Design review of the part built by this model. Coordinates are the model's own, in mm. Round coordinates to 2 decimals unless told otherwise and drop trailing zeros. Loops run counter-clockwise (first coordinate to the right, second up) from the corner with the lowest first, then second, coordinate; pieces in that order, holes last. Notation, with made-up numbers: (-38, -10) - (-10, -10) arc R19 cw to (-10, 0) - close; hole circle Ø5 at (-3.75, 24). An arc over 180 degrees is marked (long way). Answer as CSV lines item,"result". Start each with the question number.
(1) For P1, Ø4, axis at x = -32.34, y = 13.39, coming from the -Z side, flat-tipped, find the tip position at first contact; note if it passes through.
(2) Consider section C-C (x = -10.5). Give the boundary of the cut face in (y, z).
(3) Consider section D-D (z = 13.1). Count the separate pieces of the cut face and the enclosed holes in it, and give its area (3 significant figures).
(4) Wall thickness on L1, parallel to Y at x = -0.5, z = 12.3; L2, parallel to X at y = -2, z = 12.2; L3, parallel to Y at x = -6.5, z = 12.65: over which ranges is each line inside the solid? List them lowest first.
(5) Consider section A-A (x = 0). Give the boundary of the cut face in (y, z), and give its area (3 significant figures).
from build123d import *

# Parameters (mm, degrees)
SKETCH_1_R          = 40
EXTRUDE_1_DEPTH     = 12
SKETCH_8_R          = 45
EXTRUDE_3_DEPTH     = 2
SKETCH_2_R          = 7.5
CUT_EXTRUDE_1_DEPTH = 66.161338231
HOLE_WIZARD_M31_D   = 3.4
HOLE_WIZARD_M32_D   = 3.4
SKETCH_10_R         = 7.5
CUT_EXTRUDE_2_DEPTH = 66.161338231
HOLE_WIZARD_M33_D   = 3.4
SKETCH_17_R         = 17
CUT_EXTRUDE_3_DEPTH = 1.5
SKETCH_18_R         = 44.163841719
CUT_EXTRUDE_4_DEPTH = 12
SKETCH_19_R         = 17.5
CUT_EXTRUDE_5_DEPTH = 64.671029519


with BuildPart() as part:
    # Эскиз1 → Бобышка-Вытянуть1 (new body)
    with BuildSketch(Plane.XY):
        Circle(SKETCH_1_R)
    extrude(amount=EXTRUDE_1_DEPTH)

    # Эскиз8 → Бобышка-Вытянуть3 (add)
    with BuildSketch(Plane.XY.offset(12)):
        Circle(SKETCH_8_R)
    extrude(amount=EXTRUDE_3_DEPTH)

    # Эскиз2 → Вырез-Вытянуть1 (cut, through all)
    with BuildSketch(Plane(origin=(0, 0, 14), x_dir=(-1, 0, 0), z_dir=(0, 0, -1))):
        Circle(SKETCH_2_R)
    extrude(amount=CUT_EXTRUDE_1_DEPTH, mode=Mode.SUBTRACT)

    # Отверстие с зазором M31 (through all)
    with Locations(Plane(origin=(-6.663493146, -3.889871465, 14), x_dir=(-1, 0, 0), z_dir=(0, 0, 1))):
        with Locations((20.599623529, -37.010635762)):
            Hole(HOLE_WIZARD_M31_D / 2)

    # Отверстие с зазором M32 (through all)
    with Locations(Plane.XY.offset(14)):
        with Locations((0, 12.5), (-12.5, 0), (0, -12.5), (12.5, 0)):
            Hole(HOLE_WIZARD_M32_D / 2)

    # Эскиз10 → Вырез-Вытянуть2 (cut, through all)
    with BuildSketch(Plane(origin=(0, 0, 0), x_dir=(-1, 0, 0), z_dir=(0, 0, -1))):
        with Locations((0, 27.5)):
            Circle(SKETCH_10_R)
        with Locations((19.445436483, 19.445436483)):
            Circle(SKETCH_10_R)
        with Locations((27.5, 0)):
            Circle(SKETCH_10_R)
        with Locations((19.445436483, -19.445436483)):
            Circle(SKETCH_10_R)
        with Locations((0, -27.5)):
            Circle(SKETCH_10_R)
        with Locations((-19.445436483, -19.445436483)):
            Circle(SKETCH_10_R)
        with Locations((-27.5, 0)):
            Circle(SKETCH_10_R)
        with Locations((-19.445436483, 19.445436483)):
            Circle(SKETCH_10_R)
    extrude(amount=-CUT_EXTRUDE_2_DEPTH, mode=Mode.SUBTRACT)

    # Отверстие с зазором M33 (through all)
    with Locations(Plane(origin=(0, 0, 0), x_dir=(-1, 0, 0), z_dir=(0, 0, -1))):
        with Locations((-13.393920133, 32.335783638), (13.393920133, -32.335783638), (32.335783638, 13.393920133), (-32.335783638, -13.393920133)):
            Hole(HOLE_WIZARD_M33_D / 2)

    # Эскиз17 → Вырез-Вытянуть3 (cut)
    with BuildSketch(Plane(origin=(0, 0, 0), x_dir=(-1, 0, 0), z_dir=(0, 0, -1))):
        Circle(SKETCH_17_R)
    extrude(amount=-CUT_EXTRUDE_3_DEPTH, mode=Mode.SUBTRACT)

    # Эскиз18 → Вырез-Вытянуть4 (cut)
    with BuildSketch(Plane(origin=(0, 0, 0), x_dir=(-1, 0, 0), z_dir=(0, 0, -1))):
        Circle(SKETCH_18_R)
    extrude(amount=-CUT_EXTRUDE_4_DEPTH, mode=Mode.SUBTRACT)

    # Эскиз19 → Вырез-Вытянуть5 (cut, through all)
    with BuildSketch(Plane(origin=(0, 0, 12), x_dir=(-1, 0, 0), z_dir=(0, 0, -1))):
        Circle(SKETCH_19_R)
    extrude(amount=-CUT_EXTRUDE_5_DEPTH, mode=Mode.SUBTRACT)


solid = part.part
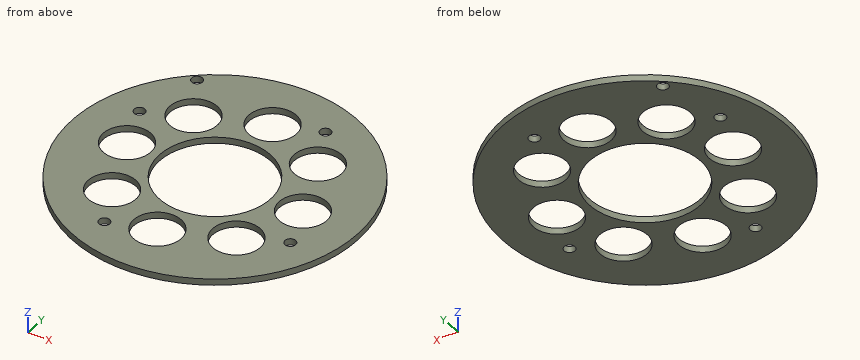
Determined:
1,P1,"stops at z = 12"
2,outline,"(-43.76, 12) - (-14, 12) - (-14, 14) - (-43.76, 14) - close; (14, 12) - (43.76, 12) - (43.76, 14) - (14, 14) - close"
3,separate pieces,"1"
3,enclosed holes,"14"
3,area,"3,940 mm^2"
4,L1,"y = -45 to -34.98, -20.02 to -17.49, 17.49 to 20.02, 34.98 to 45"
4,L2,"x = -44.96 to -34.73, -20.27 to -17.39, 17.39 to 20.27, 34.73 to 44.96"
4,L3,"y = -44.53 to -31.24, -23.76 to -16.25, 16.25 to 23.76, 31.24 to 44.53"
5,outline,"(-45, 12) - (-35, 12) - (-35, 14) - (-45, 14) - close; (-20, 12) - (-17.5, 12) - (-17.5, 14) - (-20, 14) - close; (17.5, 12) - (20, 12) - (20, 14) - (17.5, 14) - close; (35, 12) - (45, 12) - (45, 14) - (35, 14) - close"
5,area,"50.0 mm^2"
